Geometry check sheet. Reference: the model listing, model coordinates, mm. A direction names the side the tool comes from. Round coordinates to 2 decimals unless told otherwise and drop trailing zeros. Loops run counter-clockwise (first coordinate to the right, second up) from the corner with the lowest first, then second, coordinate; pieces in that order, holes last. Notation, with made-up numbers: M -22,29.25 L 9,29.25 A16 ccw 9,60.25 Z; hole C 33.5,16.5 d11. An arc over 180 degrees is marked long. Answer in a Markdown table with one row per item. Add a question column.
```python
from build123d import *

# Parameters (mm, degrees)
SCHIZZO1_R                   = 20
ESTRUSIONE_ESTRUSIONE1_DEPTH = 8
SCHIZZO2_R                   = 13.55
TAGLIO_ESTRUSIONE1_DEPTH     = 4
SCHIZZO3_W                   = 56.131286276
SCHIZZO3_H                   = 4.5
TAGLIO_ESTRUSIONE2_DEPTH     = 3.2
SCHIZZO4_R                   = 1.75
TAGLIO_ESTRUSIONE3_DEPTH     = 9


with BuildPart() as part:
    # Schizzo1 → Estrusione-Estrusione1 (new body)
    with BuildSketch(Plane(origin=(0, 0, 0), x_dir=(1, 0, 0), z_dir=(0, 1, 0))):
        Circle(SCHIZZO1_R)
    extrude(amount=ESTRUSIONE_ESTRUSIONE1_DEPTH)

    # Schizzo2 → Taglio-Estrusione1 (cut)
    with BuildSketch(Plane(origin=(0, 8, 0), x_dir=(1, 0, 0), z_dir=(0, 1, 0))):
        Circle(SCHIZZO2_R)
    extrude(amount=-TAGLIO_ESTRUSIONE1_DEPTH, mode=Mode.SUBTRACT)

    # Schizzo3 → Taglio-Estrusione2 (cut)
    with BuildSketch(Plane(origin=(0, 8, 0), x_dir=(1, 0, 0), z_dir=(0, 1, 0))):
        Rectangle(SCHIZZO3_W, SCHIZZO3_H)
    extrude(amount=-TAGLIO_ESTRUSIONE2_DEPTH, mode=Mode.SUBTRACT)

    # Schizzo4 → Taglio-Estrusione3 (cut, through all)
    with BuildSketch(Plane.XZ):
        Circle(SCHIZZO4_R)
    extrude(amount=-TAGLIO_ESTRUSIONE3_DEPTH, mode=Mode.SUBTRACT)


solid = part.part
```
1) Cross-section at B-B, the plane x = 0. Record the boundary of the cut face in (y, z).
2) Cross-section at D-D, the plane x = 16. Record the boundary of the cut face in (y, z).
3) Set-up check for faces 1 (the flat face through (3, 4, 0)), 2 (the flat face through (-17, 6, -2.25)), 3 (the flat face through (0, 8, -15)): record each of +Z, -Z, +X, -X, +Y, -Y from which the full face is reachable in a straight line by a thin tool's end or side.
4) Cross-section at A-A, the plane z = 0. Record the boundary of the cut face in (x, y), plus the area to 3 significant figures.
5) Draft check along X on faces 4 (the cylindrical face through (19.076, 3.944, -6.007)), 5 (the cylindrical face through (12.517, 6.028, 5.19)), 6 (the flat face through (17, 6, 2.25)). Enter one of: +X half, -X half, draft (parallel to the pull), parting line (faces both ways), or undercut.
6) Cross-section at C-C, the plane y = 7.5. Record the boundary of the cut face in (x, z).
7) Go/stop test with flat-tipped pins: pin 1 (4 mm diameter, centred on x = 0, z = 0, fed in from +Y); pin 2 (3 mm diameter, centred on y = 2.5, z = 6.5, fed in from -X); pin 3 (1.6 mm diameter, centred on x = 16.5, y = 7, fed in from -Z). Record where each tip stops, or that it passes through.
8) Thickness scan on L1, parallel to Z at x = 0, y = 0.9; L2, parallel to Z at x = 0, y = 7; L3, parallel to Y at x = 6, z = -5.5. Record the ranges inside material, lowest first. Write a range as [from, to].
Worked answers:
| question | item | result |
|---|---|---|
| 1 | outline | M 0,-20 L 8,-20 L 8,-13.55 L 4,-13.55 L 4,-1.75 L 0,-1.75 Z; M 0,1.75 L 4,1.75 L 4,13.55 L 8,13.55 L 8,20 L 0,20 Z |
| 2 | outline | M 0,-12 L 8,-12 L 8,-2.25 L 4.8,-2.25 L 4.8,2.25 L 8,2.25 L 8,12 L 0,12 Z |
| 3 | face 1 | +Y |
| 3 | face 2 | +X, -X, +Y |
| 3 | face 3 | +Z, -Z, +X, -X, +Y |
| 4 | outline | M -20,0 L -1.75,0 L -1.75,4 L -13.55,4 L -13.55,4.8 L -20,4.8 Z; M 1.75,0 L 20,0 L 20,4.8 L 13.55,4.8 L 13.55,4 L 1.75,4 Z |
| 4 | area | 156 mm2 |
| 5 | face 4 | parting line |
| 5 | face 5 | undercut |
| 5 | face 6 | draft |
| 6 | outline | M -19.87,-2.25 A20 ccw 19.87,-2.25 L 13.36,-2.25 A13.55 cw -13.36,-2.25 Z; M -19.87,2.25 L -13.36,2.25 A13.55 cw 13.36,2.25 L 19.87,2.25 A20 ccw Z |
| 7 | pin 1 | stops at y = 4 |
| 7 | pin 2 | stops at x = -19.36 |
| 7 | pin 3 | stops at z = -12.39 |
| 8 | L1 | z = [-20, -1.75], [1.75, 20] |
| 8 | L2 | z = [-20, -13.55], [13.55, 20] |
| 8 | L3 | y = [0, 4] |
